The model under review builds one solid part; all positions refer to its coordinate system, in mm. A direction names the side the tool comes from. Coordinates: 2 decimals unless noted, no trailing zeros. Order: outer loops, then holes, each group sorted by start corner. A loop starts at its lowest first (then second) coordinate and runs counter-clockwise, first axis right, second up. Notation, with made-up numbers: M -20,0 L 15,0 A29 ccw 15,31 Z; hole C 75,-19.5 d4. An arc over 180 degrees is marked long. Answer in a Markdown table with one row per item.
Autodesk Inventor part; units mm, degrees
ref_plane "YZ Plane" through (0, 0, 0) normal (1, 0, 0) x (0, 1, 0)
ref_plane "XZ Plane" through (0, 0, 0) normal (0, 1, 0) x (-1, 0, 0)
ref_plane "XY Plane" through (0, 0, 0) normal (0, 0, 1) x (1, 0, 0)
sketch "草圖1" plane through (0, 0, 0) normal (0, 0, 1) x (1, 0, 0)
  line L0 (0, 0) -> (-27.453, 15.85) construction
  line L1 (0, 0) -> (0, -31.7) construction
  circle A0 centre (27.453, 15.85) radius 4.5
  circle A1 centre (0, -31.7) radius 4.5
  circle A2 centre (-27.453, 15.85) radius 4.5
  line L2 (-21.703, 25.8093) -> (-5.0753, 16.2093)
  arc A3 (-5.0753, 16.2093) -> (5.0753, 16.2093) centre (0, 25) ccw
  line L3 (5.0753, 16.2093) -> (21.703, 25.8093)
  line L4 (21.703, 25.8093) -> (21.703, 25.8093)
  arc A4 (33.203, 5.8907) -> (21.703, 25.8093) centre (27.453, 15.85) ccw
  line L5 (33.203, 5.8907) -> (16.5753, -3.7093)
  arc A5 (16.5753, -3.7093) -> (11.5, -12.5) centre (21.6506, -12.5) ccw
  line L6 (11.5, -12.5) -> (11.5, -31.7)
  arc A6 (-11.5, -31.7) -> (11.5, -31.7) centre (0, -31.7) ccw
  line L7 (-11.5, -31.7) -> (-11.5, -12.5)
  arc A7 (-11.5, -12.5) -> (-16.5753, -3.7093) centre (-21.6506, -12.5) ccw
  line L8 (-16.5753, -3.7093) -> (-33.203, 5.8907)
  arc A8 (-21.703, 25.8093) -> (-33.203, 5.8907) centre (-27.453, 15.85) ccw
  line L9 (0, 0) -> (27.453, 15.85) construction
  circle A9 centre (0, 0) radius 8
  dimension "d0" = 31.7
  dimension "d4" = 120
  dimension "d5" = 31.7
  dimension "d6" = 9
  dimension "d7" = 9
  dimension "d8" = 9
  dimension "d9" = 7
  dimension "d10" = 7
  dimension "d11" = 7
  dimension "d12" = 31.7
  dimension "d13" = 120
  dimension "d35" = 25
  dimension "d38" = 16
extrude "擠出1" add sketch "草圖1" along normal blind 10 contours L2 A3 L3 A4 L5 A5 L6 A6 L7 A7 L8 A8 | A9
sketch "草圖2" plane through (0, 0, 10) normal (0, 0, 1) x (1, 0, 0)
  circle A0 centre (0, 0) radius 5
  circle A1 centre (0, 0) radius 9
  line L0 (-2.5, -6.3301) -> (2.5, -6.3301)
  line L1 (-2.5, -6.3301) -> (-2.5, -4.3301)
  line L2 (2.5, -6.3301) -> (2.5, -4.3301)
  dimension "d41" = 10
  dimension "d42" = 18
  dimension "d45" = 5
  dimension "d46" = 2
extrude "擠出2" cut sketch "草圖2" against normal through all contours A0 | A0 L2 L0 L1
extrude "擠出3" add sketch "草圖2" along normal blind 5
equation "\"d0\" = d5"
equation "\"d6\" = d8"
equation "\"d7\" = d8"
equation "\"d10\" = d9"
equation "\"d11\" = d9"
equation "\"d12\" = d5"
properties part number "carrier2"
(1) The part is to be moulded in two halves that separate along Y. For faces 4 (the cylindrical face through (0, 5, 7)), 5 (the flat face through (11.5, -22, 5)), 6 (the cylindrical face through (-12.897, -7.36, 4.93)), say which applies: +Y half, -Y half, draft (parallel to the pull), parting line (faces both ways), or undercut.
Report:
| item | result |
|---|---|
| face 4 | undercut |
| face 5 | draft |
| face 6 | -Y half |
(2) Take a section at B-B (y = 0). Write out the cut boundary in (x, z), then the cut area to 3 significant figures.
Report:
| item | result |
|---|---|
| outline | M -23,0 L -5,0 L -5,15 L -9,15 L -9,10 L -23,10 Z; M 5,0 L 23,0 L 23,10 L 9,10 L 9,15 L 5,15 Z |
| area | 400 mm^2 |
(3) Take a section at A-A (x = 0). Write out the cut boundary in (y, z).
Report:
| item | result |
|---|---|
| outline | M -43.2,0 L -36.2,0 L -36.2,10 L -43.2,10 Z; M -27.2,0 L -6.33,0 L -6.33,15 L -9,15 L -9,10 L -27.2,10 Z; M 5,0 L 14.85,0 L 14.85,10 L 9,10 L 9,15 L 5,15 Z |
(4) To check wall thickness, follow line 1 (Y direction, x = 0, z = 8.25); line 2 (Z direction, x = -11, y = 4); line 3 (X direction, y = -1.5, z = 2.5). State the ranges of each line that lie inside material, in increasing order. Write a range as [from, to].
Report:
| item | result |
|---|---|
| line 1 | [-43.2, -36.2], [-27.2, -6.33], [5, 14.85] |
| line 2 | [0, 10] |
| line 3 | [-20.4, -4.77], [4.77, 20.4] |
(5) Take a section at D-D (z = 1.5). Write out the cut boundary in (x, y).
Report:
| item | result |
|---|---|
| outline | M -33.2,5.89 L -16.58,-3.71 A10.15 cw -11.5,-12.5 L -11.5,-31.7 A11.5 ccw 11.5,-31.7 L 11.5,-12.5 A10.15 cw 16.58,-3.71 L 33.2,5.89 A11.5 ccw 21.7,25.81 L 5.08,16.21 A10.15 cw -5.08,16.21 L -21.7,25.81 A11.5 ccw Z; hole C -27.45,15.85 d9; hole C 0,-31.7 d9; hole M -2.5,-6.33 L 2.5,-6.33 L 2.5,-4.33 A5 ccw long -2.5,-4.33 Z; hole C 27.45,15.85 d9 |
(6) Machinability: for faces 1 (the cylindrical face through (-1.172, -8.923, 12.465)), 2 (the flat face through (13.27, 20.94, 4.93)), 3 (the flat face through (-11.5, -22, 5)), which of the approach directions +Z, -Z, +X, -X, +Y, -Y give a long, thin tool a straight path to every point of the face, cutting with its end or side? Answer none if there is none.
Report:
| item | result |
|---|---|
| face 1 | +Z |
| face 2 | +Z, -Z, +Y |
| face 3 | +Z, -Z, -X, -Y |
(7) Take a section at C-C (z = 13.75). Write out the cut boundary in (x, y), then the cut area to 3 significant figures.
Report:
| item | result |
|---|---|
| outline | C 0,0 d18; hole M -2.5,-6.33 L 2.5,-6.33 L 2.5,-4.33 A5 ccw long -2.5,-4.33 Z |
| area | 168 mm^2 |
(8) Insertion check: P1, Ø8, axis at x = -17, y = -9.5, coming from the -Z side; P2, Ø6, axis at x = 6, z = 4, coming from the -Y side; P3, Ø1, axis at y = -5, z = 7, coming from the -X side; P4, Ø11.5, axis at x = -27.453, y = 15.85, coming from the +Z side. Each pin has a flat end and moves straight along its axis. Give the tip position at first contact, or say it passes through.
Report:
| item | result |
|---|---|
| P1 | through |
| P2 | y = -42.8 |
| P3 | x = -15.4 |
| P4 | z = 10 |
